For this review, take the finished solid that the model builds, in its own axes (mm). A direction names the side the tool comes from. Give positions to 0.01 mm unless a question says otherwise; leave off trailing zeros. Order: outer loops, then holes, each group sorted by start corner. A loop starts at its lowest first (then second) coordinate and runs counter-clockwise, first axis right, second up. Notation, with made-up numbers: (-22, -39.5) - (2, -39.5) arc R21 cw to (2, -35.5) - close; hole circle Ø9 at (31, 42.25). An arc over 180 degrees is marked (long way). Put each result on its own line as item: value. Start each with the question number.
```python
from build123d import *

# Parameters (mm, degrees)
BOSS_EXTRUDE1_DEPTH = 40
SKETCH2_W           = 5
SKETCH2_H           = 5
CUT_EXTRUDE1_DEPTH  = 10


# Read off the part's stored shape, not the designer's step: Boss-Extrude1
with BuildPart() as part:
    # Boss-Extrude1 outline → Boss-Extrude1 (new body)
    with BuildSketch(Plane.XY):
        with BuildLine():
            Line((-5, 0), (-5, -17.588137581))
            ThreePointArc((-5, -17.588137581), (-2.5, -17.5), (0, -17.588137581))
            Line((0, -17.588137581), (0, 0))
            Line((0, 0), (-5, 0))
        make_face()
    extrude(amount=BOSS_EXTRUDE1_DEPTH)

    # Sketch2 → Cut-Extrude1 (cut)
    with BuildSketch(Plane(origin=(0, 0, 0), x_dir=(0, 0, -1), z_dir=(1, 0, 0))):
        with Locations((-2.5, -2.5)):
            Rectangle(SKETCH2_W, SKETCH2_H)
        with Locations((-17.5, 17.5)):
            Rectangle(SKETCH2_W, SKETCH2_H)
    extrude(amount=-CUT_EXTRUDE1_DEPTH, mode=Mode.SUBTRACT)


solid = part.part
```
1. Add section B-B, the plane y = -2.5. Give the boundary of the cut face in (x, z), then the cut area to 3 significant figures.
2. Add section A-A, the plane x = -2.5. Give the boundary of the cut face in (y, z), then the cut area to 3 significant figures.
3. Wall thickness on line 1 (Z direction, x = -2.9, y = -1); line 2 (Y direction, x = -2.8, z = 7); line 3 (Y direction, x = -3.8, z = 2): over which ranges is each line inside the solid? List them lowest first. Write a range as from..to.
4. Clearance check with flat-ended pins moving along their axes: pin 1 (2 mm diameter, centred on x = -2.5, y = -2, fed in from -Z); pin 2 (2.5 mm diameter, centred on x = -2.5, z = 2, fed in from +Y). State where each tip first meets the part, or that it passes through.
5. Add section C-C, the plane x = -0.45. Give the boundary of the cut face in (y, z), then the cut area to 3 significant figures.
6. Tool access review of faces 1 (the face through (-3, -9, 40)), 2 (the face through (-2, -5, 3)): name each direction out of +Z, -Z, +X, -X, +Y, -Y from which nothing blocks a thin tool from reaching the whole face with its end or side.
Found:
1. outline: (-5, 5) - (0, 5) - (0, 40) - (-5, 40) - close
1. area: 175 mm^2
2. outline: (-17.5, 0) - (-5, 0) - (-5, 5) - (0, 5) - (0, 40) - (-17.5, 40) - close
2. area: 675 mm^2
3. line 1: z = 5..40
3. line 2: y = -17.5..0
3. line 3: y = -17.52..-5
4. pin 1: stops at z = 5
4. pin 2: stops at y = -5
5. outline: (-17.56, 0) - (-5, 0) - (-5, 5) - (0, 5) - (0, 40) - (-17.56, 40) - close
5. area: 677 mm^2
6. face 1: +Z, +X, -X, +Y, -Y
6. face 2: -Z, +X, -X, +Y
